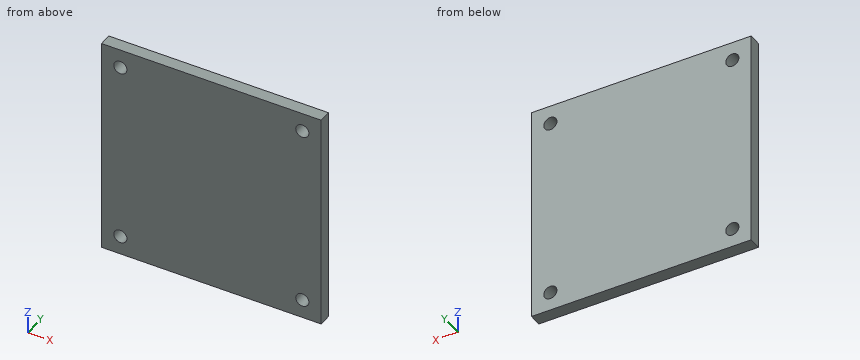
Autodesk Inventor part; units mm, degrees
ref_plane "YZ Plane" through (0, 0, 0) normal (1, 0, 0) x (0, 1, 0)
ref_plane "XZ Plane" through (0, 0, 0) normal (0, 1, 0) x (-1, 0, 0)
ref_plane "XY Plane" through (0, 0, 0) normal (0, 0, 1) x (1, 0, 0)
sketch "草图1" plane through (0, 0, 0) normal (0, 1, 0) x (-1, 0, 0)
  line L0 (0, 0) -> (-35, 0)
  line L1 (-35, 0) -> (-35, -35)
  line L2 (-35, -35) -> (0, -35)
  line L3 (0, -35) -> (0, 0)
  circle A0 centre (-3, -3) radius 1.05
  line L4 (0, -17.5) -> (-35, -17.5)
  line L5 (-17.5, 0) -> (-17.5, -35)
  circle A1 centre (-3, -32) radius 1.05
  circle A2 centre (-32, -3) radius 1.05
  circle A3 centre (-32, -32) radius 1.05
  dimension "d0" = 35
  dimension "d1" = 35
  dimension "d2" = 2.1
  dimension "d6" = 3
  dimension "d7" = 3
extrude "拉伸1" add sketch "草图1" along normal blind 2
properties part number "飞控外壳"
The model under review builds one solid part; all positions refer to its coordinate system, in mm. Round coordinates to 2 decimals unless told otherwise and drop trailing zeros. Write each loop counter-clockwise with the first axis right and the second up, starting at its lowest first coordinate (ties: lowest second). Pieces come first, ordered by that corner, then holes. Notation, with made-up numbers: (36, 34) - (61, 34) arc R23 cw to (61, 65) - close; hole circle Ø4 at (30, 20.25). An arc over 180 degrees is marked (long way). Answer as CSV lines item,"result". Start each with the question number.
(1) To check wall thickness, follow line 1 (Z direction, x = 32, y = 1.1); line 2 (Z direction, x = 3.5, y = 1.3). State the ranges of each line that lie inside material, in increasing order.
(2) We need section A-A on z = -3. State the section outline as (x, y) points, plus the area to 3 significant figures.
(3) We need section B-B on x = 32. State the section outline as (y, z) points, plus the area to 3 significant figures.
Worked answers:
1,line 1,"-35 to -33.05, -30.95 to -4.05, -1.95 to 0"
1,line 2,"-35 to -32.92, -31.08 to -3.92, -2.08 to 0"
2,outline,"(0, 0) - (1.95, 0) - (1.95, 2) - (0, 2) - close; (4.05, 0) - (30.95, 0) - (30.95, 2) - (4.05, 2) - close; (33.05, 0) - (35, 0) - (35, 2) - (33.05, 2) - close"
2,area,"61.6 mm²"
3,outline,"(0, -35) - (2, -35) - (2, -33.05) - (0, -33.05) - close; (0, -30.95) - (2, -30.95) - (2, -4.05) - (0, -4.05) - close; (0, -1.95) - (2, -1.95) - (2, 0) - (0, 0) - close"
3,area,"61.6 mm²"
